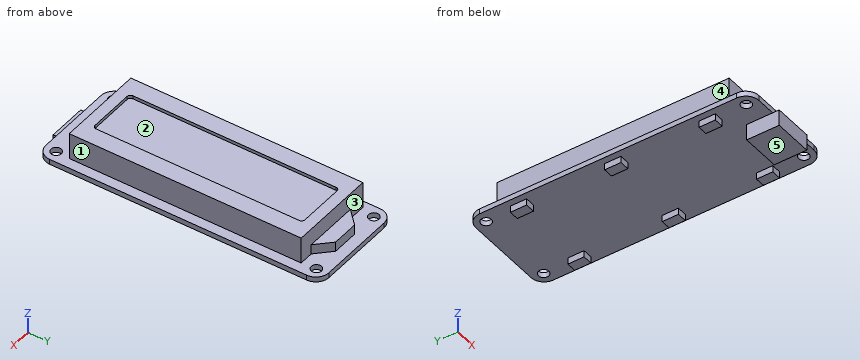
Autodesk Fusion 360 part; units mm, degrees
sketch "Skizze1" plane through (0, 0, 0) normal (0, 0, 1) x (1, 0, 0)
  line L0 (4, 0) -> (28, 0)
  line L1 (32, 4) -> (32, 83)
  line L2 (28, 87) -> (4, 87)
  line L3 (0, 83) -> (0, 4)
  circle A0 centre (3.5, 3.5) radius 1.6
  circle A1 centre (28.5, 3.5) radius 1.6
  circle A2 centre (3.5, 83.5) radius 1.6
  circle A3 centre (28.5, 83.5) radius 1.6
  arc A4 (4, 87) -> (0, 83) centre (4, 83) ccw
  arc A5 (32, 83) -> (28, 87) centre (28, 83) ccw
  arc A6 (0, 4) -> (4, 0) centre (4, 4) ccw
  arc A7 (28, 0) -> (32, 4) centre (28, 4) ccw
  point P0 (32, 0)
  point P1 (0, 87)
  dimension "d1" = 32
  dimension "d2" = 87
  dimension "d3" = 3.2
  dimension "d4" = 3.5
  dimension "d5" = 3.5
  dimension "d8" = 25
  dimension "d9" = 80
  dimension "d10" = 4
extrude "Extrusion1" add sketch "Skizze1" along normal blind 1.6
sketch "Skizze2" plane through (0, 0, 1.6) normal (0, 0, 1) x (-1, 0, 0)
  circle A0 centre (-28.5, -3.5) radius 1.6
  circle A1 centre (-3.5, -3.5) radius 1.6
  circle A2 centre (-3.5, -83.5) radius 1.6
  circle A3 centre (-28.5, -83.5) radius 1.6
  arc A4 (-28, 0) -> (-32, -4) centre (-28, -4) ccw
  line L0 (-32, -4) -> (-32, -83)
  arc A5 (-32, -83) -> (-28, -87) centre (-28, -83) ccw
  line L1 (-28, -87) -> (-4, -87)
  arc A6 (-4, -87) -> (0, -83) centre (-4, -83) ccw
  line L2 (0, -83) -> (0, -4)
  arc A7 (0, -4) -> (-4, 0) centre (-4, -4) ccw
  line L3 (-4, 0) -> (-28, 0)
  line L4 (-2.08, -7.8) -> (-28.88, -7.8)
  line L5 (-28.88, -7.8) -> (-28.88, -79.1)
  line L6 (-28.88, -79.1) -> (-2.08, -79.1)
  line L7 (-2.08, -79.1) -> (-2.08, -7.8)
  dimension "d13" = 26.8
  dimension "d14" = 71.3
  dimension "d15" = 7.8
  dimension "d16" = 2.08
extrude "Extrusion2" add sketch "Skizze2" along normal blind 8.1 contours L4 L5 L6 L7
sketch "Skizze3" plane through (0, 0, 9.7) normal (0, 0, 1) x (-1, 0, 0)
  line L0 (-2.08, -79.1) -> (-2.08, -7.8)
  line L1 (-2.08, -7.8) -> (-28.88, -7.8)
  line L2 (-28.88, -7.8) -> (-28.88, -79.1)
  line L3 (-28.88, -79.1) -> (-2.08, -79.1)
  line L4 (-8.48, -11.2) -> (-22.48, -11.2)
  line L5 (-23.48, -12.2) -> (-23.48, -74.7)
  line L6 (-22.48, -75.7) -> (-8.48, -75.7)
  line L7 (-7.48, -74.7) -> (-7.48, -12.2)
  arc A0 (-7.48, -12.2) -> (-8.48, -11.2) centre (-8.48, -12.2) ccw
  arc A1 (-22.48, -11.2) -> (-23.48, -12.2) centre (-22.48, -12.2) ccw
  arc A2 (-8.48, -75.7) -> (-7.48, -74.7) centre (-8.48, -74.7) ccw
  arc A3 (-23.48, -74.7) -> (-22.48, -75.7) centre (-22.48, -74.7) ccw
  point P0 (-7.48, -11.2)
  point P1 (-23.48, -11.2)
  point P2 (-7.48, -75.7)
  dimension "d19" = 16
  dimension "d20" = 64.5
  dimension "d21" = 3.4
  dimension "d22" = 5.4
  dimension "d23" = 1
extrude "Extrusion3" cut sketch "Skizze3" against normal blind 1 contours L4 L5 L6 L7 A0 A1 A2 A3
sketch "Skizze4" plane through (0, 0, 1.6) normal (0, 0, 1) x (-1, 0, 0)
  line L0 (-2.08, -79.1) -> (-28.88, -79.1)
  line L1 (-28.88, -79.1) -> (-28.88, -7.8)
  line L2 (-28.88, -7.8) -> (-2.08, -7.8)
  line L3 (-2.08, -7.8) -> (-2.08, -79.1)
  circle A0 centre (-28.5, -3.5) radius 1.6
  circle A1 centre (-3.5, -3.5) radius 1.6
  circle A2 centre (-3.5, -83.5) radius 1.6
  circle A3 centre (-28.5, -83.5) radius 1.6
  arc A4 (-28, 0) -> (-32, -4) centre (-28, -4) ccw
  line L4 (-32, -4) -> (-32, -83)
  arc A5 (-32, -83) -> (-28, -87) centre (-28, -83) ccw
  line L5 (-28, -87) -> (-4, -87)
  arc A6 (-4, -87) -> (0, -83) centre (-4, -83) ccw
  line L6 (0, -83) -> (0, -4)
  arc A7 (0, -4) -> (-4, 0) centre (-4, -4) ccw
  line L7 (-4, 0) -> (-28, 0)
  line L8 (-7.48, -79.1) -> (-11.88, -83.5)
  line L9 (-11.88, -83.5) -> (-20.12, -83.5)
  line L10 (-20.12, -83.5) -> (-24.52, -79.1)
  dimension "d26" = 7.48
  dimension "d27" = 7.48
  dimension "d28" = 3.5
  dimension "d29" = 45
  dimension "d30" = 45
extrude "Extrusion4" add sketch "Skizze4" along normal blind 3 contours L0 L8 L9 L10
sketch "Skizze5" plane through (0, 0, 0) normal (0, 0, -1) x (1, 0, 0)
  circle A0 centre (28.5, -3.5) radius 1.6
  circle A1 centre (3.5, -3.5) radius 1.6
  circle A2 centre (3.5, -83.5) radius 1.6
  circle A3 centre (28.5, -83.5) radius 1.6
  arc A4 (32, -4) -> (28, 0) centre (28, -4) ccw
  line L0 (28, 0) -> (4, 0)
  arc A5 (4, 0) -> (0, -4) centre (4, -4) ccw
  line L1 (0, -4) -> (0, -83)
  arc A6 (0, -83) -> (4, -87) centre (4, -83) ccw
  line L2 (4, -87) -> (28, -87)
  arc A7 (28, -87) -> (32, -83) centre (28, -83) ccw
  line L3 (32, -83) -> (32, -4)
  line L4 (2, -12) -> (5, -12)
  line L5 (5, -12) -> (5, -17)
  line L6 (5, -17) -> (2, -17)
  line L7 (2, -17) -> (2, -12)
  line L8 (30, -12) -> (30, -17)
  line L9 (30, -17) -> (27, -17)
  line L10 (27, -12) -> (30, -12)
  line L11 (27, -17) -> (27, -12)
  line L12 (5, -41) -> (5, -46)
  line L13 (5, -46) -> (2, -46)
  line L14 (2, -41) -> (5, -41)
  line L15 (2, -46) -> (2, -41)
  line L16 (30, -41) -> (30, -46)
  line L17 (30, -46) -> (27, -46)
  line L18 (27, -41) -> (30, -41)
  line L19 (27, -46) -> (27, -41)
  line L20 (5, -70) -> (5, -75)
  line L21 (5, -75) -> (2, -75)
  line L22 (2, -70) -> (5, -70)
  line L23 (2, -75) -> (2, -70)
  line L24 (30, -70) -> (30, -75)
  line L25 (30, -75) -> (27, -75)
  line L26 (27, -70) -> (30, -70)
  line L27 (27, -75) -> (27, -70)
  dimension "d33" = 3
  dimension "d34" = 5
  dimension "d35" = 12
  dimension "d36" = 2
  dimension "d39" = 25
  dimension "d40" = -58
extrude "Extrusion5" add sketch "Skizze5" along normal blind 2 contours L4 L5 L6 L7 | L8 L9 L10 L11 | L12 L13 L14 L15 | L16 L17 L18 L19 | L20 L21 L22 L23 | L24 L25 L26 L27
sketch "Skizze6" plane through (0, 0, 0) normal (0, 0, -1) x (1, 0, 0)
  line L0 (2, -17) -> (2, -12)
  line L1 (2, -12) -> (5, -12)
  line L2 (5, -12) -> (5, -17)
  line L3 (5, -17) -> (2, -17)
  line L4 (2, -75) -> (2, -70)
  line L5 (2, -70) -> (5, -70)
  line L6 (5, -70) -> (5, -75)
  line L7 (5, -75) -> (2, -75)
  line L8 (2, -46) -> (2, -41)
  line L9 (2, -41) -> (5, -41)
  line L10 (5, -41) -> (5, -46)
  line L11 (5, -46) -> (2, -46)
  line L12 (27, -17) -> (27, -12)
  line L13 (27, -12) -> (30, -12)
  line L14 (30, -12) -> (30, -17)
  line L15 (30, -17) -> (27, -17)
  line L16 (27, -75) -> (27, -70)
  line L17 (27, -70) -> (30, -70)
  line L18 (30, -70) -> (30, -75)
  line L19 (30, -75) -> (27, -75)
  line L20 (27, -46) -> (27, -41)
  line L21 (27, -41) -> (30, -41)
  line L22 (30, -41) -> (30, -46)
  line L23 (30, -46) -> (27, -46)
  circle A0 centre (28.5, -3.5) radius 1.6
  circle A1 centre (3.5, -3.5) radius 1.6
  circle A2 centre (3.5, -83.5) radius 1.6
  circle A3 centre (28.5, -83.5) radius 1.6
  arc A4 (32, -4) -> (28, 0) centre (28, -4) ccw
  line L24 (28, 0) -> (4, 0)
  arc A5 (4, 0) -> (0, -4) centre (4, -4) ccw
  line L25 (0, -4) -> (0, -83)
  arc A6 (0, -83) -> (4, -87) centre (4, -83) ccw
  line L26 (4, -87) -> (28, -87)
  arc A7 (28, -87) -> (32, -83) centre (28, -83) ccw
  line L27 (32, -83) -> (32, -4)
  line L28 (10, 2) -> (22, 2)
  line L29 (22, 2) -> (22, -8)
  line L30 (22, -8) -> (10, -8)
  line L31 (10, -8) -> (10, 2)
  dimension "d43" = 12
  dimension "d44" = 10
  dimension "d45" = 2
  dimension "d46" = 10
extrude "Extrusion6" add sketch "Skizze6" along normal blind 5 contours L24 L29 L30 L31 | L24 L28 L29 L31
Source: CAD feature listing. Evaluate the final solid. Frame: model axes, mm. Face numbers are marked on the shaded views. A direction names the side the tool comes from. Give positions to 0.01 mm unless a question says otherwise; leave off trailing zeros. Loops run counter-clockwise (first coordinate to the right, second up) from the corner with the lowest first, then second, coordinate; pieces in that order, holes last. Notation, with made-up numbers: (88, 81.5) -> (109, 81.5) arc R16 ccw to (109, 106.5) -> close; hole circle Ø1 at (30.5, 28). An arc over 180 degrees is marked (long way). Use a Markdown table: item, result. Add a question column.
(1) Section query A-A (y = 9). Output: boundary loops of the cut face in (x, z), then the cut area to 3 significant figures.
(2) First-contact query: pin 1 Ø1 at (y, z) = (31.5, 5.5) entering from +X; pin 2 Ø2 at (x, z) = (3.5, -1.5) entering from -Y; pin 3 Ø4 at (y, z) = (58, 5.5) entering from -X. Flat tips, straight axial feed; report the tip coordinate or a pass-through.
(3) Ray query, line 1 (Y direction, x = 3.5, z = 0.4); line 2 (X direction, y = 83.5, z = 1.05); line 3 (Y direction, x = 15, z = 0.5). Return the intervals inside material, ascending.
(4) Section query B-B (z = 3). Output: boundary loops of the cut face in (x, y).
(5) Section query C-C (x = 3). Output: boundary loops of the cut face in (y, z).
(6) Access query for the marked faces 4 and 5. Directions: +Z, -Z, +X, -X, +Y, -Y. A direction counts if a zero-diameter tool reaches every point of the face in a straight line with its end or side. Return the directions, or none.
(7) Section query D-D (z = -3). Output: boundary loops of the cut face in (x, y), then the cut area to 3 significant figures.
(8) Pull-direction query (Y, two-part tool) for the marked faces 1, 2 and 3; classes: +Y half, -Y half, draft (parallel to the pull), parting line (faces both ways), or undercut.
Checked values:
| question | item | result |
|---|---|---|
| 1 | outline | (0, 0) -> (32, 0) -> (32, 1.6) -> (28.88, 1.6) -> (28.88, 9.7) -> (2.08, 9.7) -> (2.08, 1.6) -> (0, 1.6) -> close |
| 1 | area | 268 mm^2 |
| 2 | pin 1 | x = 28.88 |
| 2 | pin 2 | y = 12 |
| 2 | pin 3 | x = 2.08 |
| 3 | line 1 | 0.03 to 1.9, 5.1 to 81.9, 85.1 to 86.97 |
| 3 | line 2 | 0.03 to 1.9, 5.1 to 26.9, 30.1 to 31.97 |
| 3 | line 3 | 0 to 87 |
| 4 | outline | (2.08, 7.8) -> (28.88, 7.8) -> (28.88, 79.1) -> (24.52, 79.1) -> (20.12, 83.5) -> (11.88, 83.5) -> (7.48, 79.1) -> (2.08, 79.1) -> close |
| 5 | outline | (0.13, 0) -> (1.98, 0) -> (1.98, 1.6) -> (0.13, 1.6) -> close; (5.02, 0) -> (12, 0) -> (12, -2) -> (17, -2) -> (17, 0) -> (41, 0) -> (41, -2) -> (46, -2) -> (46, 0) -> (70, 0) -> (70, -2) -> (75, -2) -> (75, 0) -> (81.98, 0) -> (81.98, 1.6) -> (79.1, 1.6) -> (79.1, 9.7) -> (7.8, 9.7) -> (7.8, 1.6) -> (5.02, 1.6) -> close; (85.02, 0) -> (86.87, 0) -> (86.87, 1.6) -> (85.02, 1.6) -> close |
| 6 | face 4 | +Z, -X, +Y, -Y |
| 6 | face 5 | -Z, +X, -X, +Y, -Y |
| 7 | outline | (10, -2) -> (22, -2) -> (22, 8) -> (10, 8) -> close |
| 7 | area | 120 mm^2 |
| 8 | face 1 | draft |
| 8 | face 2 | undercut |
| 8 | face 3 | +Y half |
